from build123d import *

# Parameters (mm, degrees)
F0_R     = 16.75
F0_R_2   = 1.25
F1_DEPTH = 4.5
F0_R_3   = 17.75
F2_DEPTH = 1


# Not quite as in the source:
# - a feature names something its author has since deleted; it is built from what else it names


with BuildPart() as f1:
    # F0 (on Top) → F1 (new body)
    with BuildSketch(Plane.XY):
        Circle(F0_R)
        with BuildLine():
            ThreePointArc((1.9843134833, 2.25), (2.7343134833, 1.2343134833), (3, 0))
            ThreePointArc((3, 0), (-1.2343134833, -2.7343134833), (-1.9843134833, 2.25))
            Line((-1.9843134833, 2.25), (-2, 2.25))
            Line((-2, 2.25), (-2, 5.25))
            Line((-2, 5.25), (2, 5.25))
            Line((2, 5.25), (2, 2.25))
            Line((2, 2.25), (1.9843134833, 2.25))
        make_face(mode=Mode.SUBTRACT)
        with Locations((0, 11.9703095406)):
            Circle(F0_R_2, mode=Mode.SUBTRACT)
    extrude(amount=F1_DEPTH)

    # F0 (on Top) → F2 (join)
    with BuildSketch(Plane.XY):
        Circle(F0_R_3)
        Circle(F0_R, mode=Mode.SUBTRACT)
    extrude(amount=F2_DEPTH)


solid = f1.part
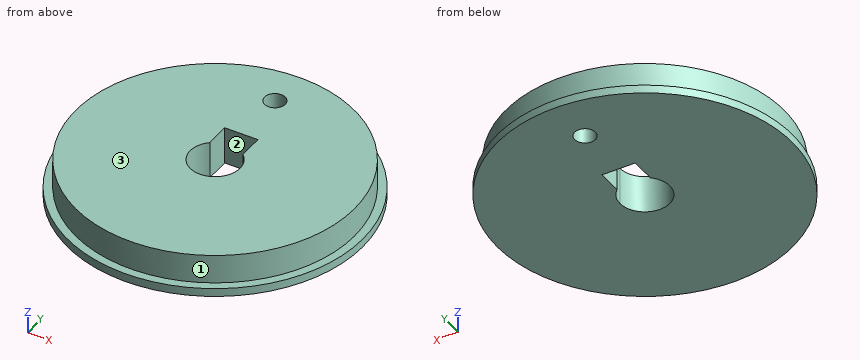
Here's how the part is built. I have some questions about the finished solid (model axes, mm). Face numbers are marked on the shaded views. Round coordinates to 2 decimals unless told otherwise and drop trailing zeros. Write each loop counter-clockwise with the first axis right and the second up, starting at its lowest first coordinate (ties: lowest second). Pieces come first, ordered by that corner, then holes.
1. If we mould it in two halves opening along Y, with no side actions, what happens to the marked faces 1, 2 and 3? For each: released by +Y, released by -Y, zero draft, split by the parting line, or undercut.
2. Suppose I cut it at D-D (y = 8.5). List the corners of the cut face in (x, z) for me.
3. Suppose I cut it at A-A (x = 0). List the corners of the cut face in (y, z) for me, and give its area (3 significant figures).
4. Suppose I cut it at C-C (y = 3). List the corners of the cut face in (x, z) for me, and give its area (3 significant figures).
5. Will this pin go through, and if not, where does the flat tip stop? pin 1 Ø2 at (x, z) = (-0.5, 2.5) entering from -Y.
6. I need wall thicknesses on L1, parallel to Y at x = 0, z = 3.4; L2, parallel to Z at x = 6.5, y = 15.5; L3, parallel to X at y = 4, z = 2.35. Which ranges of each line are inside material? Lowest first, please.
7. Suppose I cut it at B-B (z = 1.9). State how many separate pieces and enclosed holes the cut face has, and give its area (3 significant figures).
Answer sheet:
1. face 1: split by the parting line
1. face 2: undercut
1. face 3: zero draft
2. outline: (-15.58, 0) - (15.58, 0) - (15.58, 1) - (14.43, 1) - (14.43, 4.5) - (-14.43, 4.5) - (-14.43, 1) - (-15.58, 1) - close
3. outline: (-17.75, 0) - (-3, 0) - (-3, 4.5) - (-16.75, 4.5) - (-16.75, 1) - (-17.75, 1) - close; (5.25, 0) - (10.72, 0) - (10.72, 4.5) - (5.25, 4.5) - close; (13.22, 0) - (17.75, 0) - (17.75, 1) - (16.75, 1) - (16.75, 4.5) - (13.22, 4.5) - close
3. area: 104 mm2
4. outline: (-17.49, 0) - (-2, 0) - (-2, 4.5) - (-16.48, 4.5) - (-16.48, 1) - (-17.49, 1) - close; (2, 0) - (17.49, 0) - (17.49, 1) - (16.48, 1) - (16.48, 4.5) - (2, 4.5) - close
4. area: 132 mm2
5. pin 1: stops at y = -16.75
6. L1: y = -16.75 to -3, 5.25 to 10.72, 13.22 to 16.75
6. L2: z = 0 to 1
6. L3: x = -16.27 to -2, 2 to 16.27
7. separate pieces: 1
7. enclosed holes: 2
7. area: 838 mm2
